Design review of the part built by this model. Coordinates are the model's own, in mm. A direction names the side the tool comes from. Give positions to 0.01 mm unless a question says otherwise; leave off trailing zeros. Loops run counter-clockwise (first coordinate to the right, second up) from the corner with the lowest first, then second, coordinate; pieces in that order, holes last. Notation, with made-up numbers: M -40,21.25 L 9,21.25 A14 ccw 9,39.25 Z; hole C 87.5,24 d7. An arc over 180 degrees is marked long. Use a Markdown table: item, result. Add a question column.
(1) Add section C-C, the plane y = -2.25. Give the boundary of the cut face in (x, z).
(2) For probe 1 along Z at (x, y) = (-22.5, -1); probe 2 along X at (y, z) = (-1, 17.5); probe 3 along X at (y, z) = (-2.3, -26), list the stretches that pass through material, from the lowest coordinate up.
(3) For faces 1 (the face through (19, 0, -19)), 2 (the face through (-0.11, -2.1, -26.11)), list the 3-axis set-ups (+Z, -Z, +X, -X, +Y, -Y) from which the entire face can be reached by the end or side of a thin tool; tool diameter is ignored.
(4) Draft analysis for pull direction Z (two halves, no side actions). For faces 3 (the face through (29, -3, 1)), 4 (the face through (20.765, -1.479, -39.923)), 5 (the face through (-13.14, -2.1, -22.56)), state which applies: pulls with the +Z half, pulls with the -Z half, needs draft (parallel to the pull), parting line crosses it, or undercut.
(5) Add section D-D, the plane x = -38.5. Give the boundary of the cut face in (y, z), then the cut area to 3 significant figures.
```python
from build123d import *

# Parameters (mm, degrees)
F0_R     = 45
F1_DEPTH = 3
F2_R     = 2.99999


# Not quite as in the source:
# - a fillet or chamfer is up to 0.001 mm smaller than in the source, because OpenCascade refuses the exact size


with BuildPart() as f1:
    # F0 (on Front) → F1 (new body)
    with BuildSketch(Plane.XZ):
        Circle(F0_R)
        Polygon((-18.4842828911, 18.4842828911), (-6.7657171089, 25.25), (6.7657171089, 25.25), (18.4842828911, 18.4842828911), (25.25, 6.7657171089), (25.25, -6.7657171089), (18.4842828911, -18.4842828911), (6.7657171089, -25.25), (-6.7657171089, -25.25), (-18.4842828911, -18.4842828911), (-25.25, -6.7657171089), (-25.25, 6.7657171089), align=None, mode=Mode.SUBTRACT)
    extrude(amount=F1_DEPTH)

    # F2 (radius 3 in the source; OpenCascade refuses exactly that, so slightly less here)
    f2_edges = [f1.edges().sort_by_distance(p)[0] for p in [
        (-12.625, -3, 21.867141),
        (-21.867141, -3, 12.625),
        (-25.25, -3, 0),
        (-21.867141, -3, -12.625),
        (-12.625, -3, -21.867141),
        (0, -3, -25.25),
        (12.625, -3, -21.867141),
        (21.867141, -3, -12.625),
        (25.25, -3, 0),
        (21.867141, -3, 12.625),
        (12.625, -3, 21.867141),
        (0, -3, 25.25),
    ]]
    fillet(f2_edges, radius=F2_R)


solid = f1.part
```
Established:
| question | item | result |
|---|---|---|
| 1 | outline | C 0,0 d90; hole M -26.27,-7.04 L -19.23,-19.23 L -7.04,-26.27 L 7.04,-26.27 L 19.23,-19.23 L 26.27,-7.04 L 26.27,7.04 L 19.23,19.23 L 7.04,26.27 L -7.04,26.27 L -19.23,19.23 L -26.27,7.04 Z |
| 2 | probe 1 | -38.97 to -11.87, 11.87 to 38.97 |
| 2 | probe 2 | -41.46 to -19.25, 19.25 to 41.46 |
| 2 | probe 3 | -36.73 to -7.61, 7.61 to 36.73 |
| 3 | face 1 | +Z, -Z, +X, -X, +Y |
| 3 | face 2 | -Y |
| 4 | face 3 | needs draft |
| 4 | face 4 | parting line crosses it |
| 4 | face 5 | undercut |
| 5 | outline | M -3,-23.3 L 0,-23.3 L 0,23.3 L -3,23.3 Z |
| 5 | area | 140 mm^2 |
